The model under review builds one solid part; all positions refer to its coordinate system, in mm. Face numbers are marked on the shaded views. A direction names the side the tool comes from. Give positions to 0.01 mm unless a question says otherwise; leave off trailing zeros. Order: outer loops, then holes, each group sorted by start corner. A loop starts at its lowest first (then second) coordinate and runs counter-clockwise, first axis right, second up.
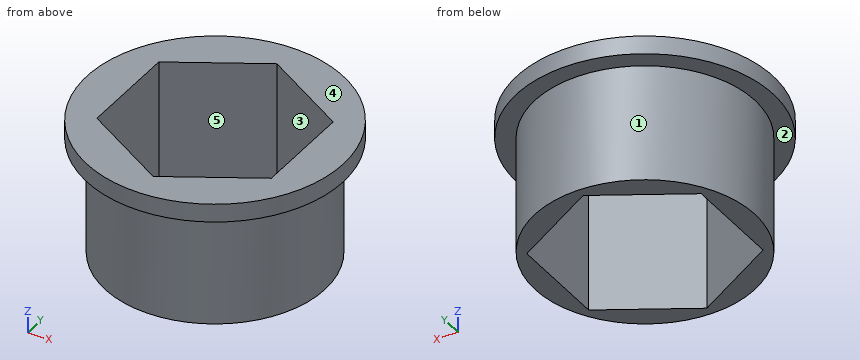
```python
from build123d import *

# Parameters (mm, degrees)
SKETCH1_R               = 12
SKETCH1_R_2             = 6.4
BOSS_EXTRUDE1_DEPTH     = 7.4
SKETCH3_R               = 14
BOSS_EXTRUDE3_DEPTH     = 2
SKETCH1_4_R             = 6.4
CUT_EXTRUDE4_DEPTH      = 22.136697945
CUT_EXTRUDE4_DEPTH_BACK = 22.136697945


with BuildPart() as part:
    # Sketch1 → Boss-Extrude1 (new, symmetric)
    with BuildSketch(Plane.XY):
        Circle(SKETCH1_R)
        Circle(SKETCH1_R_2, mode=Mode.SUBTRACT)
    extrude(amount=BOSS_EXTRUDE1_DEPTH, both=True)

    # Sketch3 → Boss-Extrude3 (add)
    with BuildSketch(Plane.XY.offset(7.4)):
        Circle(SKETCH3_R)
    extrude(amount=-BOSS_EXTRUDE3_DEPTH)

    # Sketch1_4 → Cut-Extrude4 (cut, two sides)
    with BuildSketch(Plane.XY) as cut_extrude4_sk:
        Polygon((-9.526279442, 5.5), (-9.526279442, -5.5), (0, -11), (9.526279442, -5.5), (9.526279442, 5.5), (0, 11), align=None)
        Circle(SKETCH1_4_R, mode=Mode.SUBTRACT)
        Circle(SKETCH1_4_R)
    extrude(amount=CUT_EXTRUDE4_DEPTH, mode=Mode.SUBTRACT)
    extrude(cut_extrude4_sk.sketch, amount=-CUT_EXTRUDE4_DEPTH_BACK, mode=Mode.SUBTRACT)


solid = part.part
```
Item 1: Take a section at C-C (x = -5.75). Give the boundary of the cut face in (y, z), and give its area (3 significant figures).
Values found:
outline: (-12.76, 5.4) - (-10.53, 5.4) - (-10.53, -7.4) - (-7.68, -7.4) - (-7.68, 7.4) - (-12.76, 7.4) - close; (7.68, -7.4) - (10.53, -7.4) - (10.53, 5.4) - (12.76, 5.4) - (12.76, 7.4) - (7.68, 7.4) - close
area: 93.4 mm2
Item 2: Clearance check with flat-ended pins moving along their axes: pin 1 Ø2 at (y, z) = (-2, 4) entering from -X; pin 2 Ø1 at (y, z) = (-10, 0.5) entering from -X; pin 3 Ø5 at (x, z) = (-10.5, -2) entering from +Y. State where each tip first meets the part, or that it passes through.
Values found:
pin 1: stops at x = -11.96
pin 2: stops at x = -7.33
pin 3: stops at y = 8.94
Item 3: Draft analysis for pull direction X (two halves, no side actions). For the marked faces 1, 2 and 3, state which applies: released by +X, released by -X, zero draft, split by the parting line, or undercut.
Values found:
face 1: split by the parting line
face 2: zero draft
face 3: undercut
Item 4: Take a section at A-A (y = 0). Give the boundary of the cut face in (x, z).
Values found:
outline: (-14, 5.4) - (-12, 5.4) - (-12, -7.4) - (-9.53, -7.4) - (-9.53, 7.4) - (-14, 7.4) - close; (9.53, -7.4) - (12, -7.4) - (12, 5.4) - (14, 5.4) - (14, 7.4) - (9.53, 7.4) - close
Item 5: Take a section at B-B (z = 1.5). Give the boundary of the cut face in (x, y), and give its area (3 significant figures).
Values found:
outline: circle Ø24 at (0, 0); hole (-9.53, -5.5) - (0, -11) - (9.53, -5.5) - (9.53, 5.5) - (0, 11) - (-9.53, 5.5) - close
area: 138 mm2
Item 6: For line 1 (Z direction, x = 0.75, y = -12.5); line 2 (Y direction, x = 3, z = -2.75); line 3 (Y direction, x = -4.25, z = 6.5), list the stretches that pass through material, from the lowest coordinate up.
Values found:
line 1: z = 5.4 to 7.4
line 2: y = -11.62 to -9.27, 9.27 to 11.62
line 3: y = -13.34 to -8.55, 8.55 to 13.34
Item 7: For the marked faces 4 and 5, list the 3-axis set-ups (+Z, -Z, +X, -X, +Y, -Y) from which the entire face can be reached by the end or side of a thin tool; tool diameter is ignored.
Values found:
face 4: +Z, +X, -X, +Y, -Y
face 5: +Z, -Z
